Input: part model. Units: mm. Frame: model coordinates. Coordinates: 2 decimals unless noted, no trailing zeros. Write each loop counter-clockwise with the first axis right and the second up, starting at its lowest first coordinate (ties: lowest second). Pieces come first, ordered by that corner, then holes. Notation, with made-up numbers: (49, -37) -> (93, -37) arc R31 ccw to (93, -1) -> close; hole circle Ø2 at (76.5, -26). An arc over 180 degrees is marked (long way). Use one line per item in the form item = value. Start each with the question number.
(1) Cut plane C-C on y = 17. Return the cut outline in (x, z), plus the area to 3 significant figures.
(2) Cut plane A-A on x = 0. Return the cut outline in (y, z).
(3) Pull-direction query (X, two-part tool) for faces 1 (the face through (-26, 31.75, 2)), 2 (the face through (7.629, 15.653, 24.227)), 3 (the face through (10.48, 15.65, 33.29)); classes: released by +X, released by -X, zero draft, split by the parting line, or undercut.
(4) Ray query, line 1 along Y through (x, z) = (0, 28.75); line 2 along X through (y, z) = (18, -1); line 3 along X through (y, z) = (22, -17). Return the intervals inside material, ascending.
(5) Cut plane D-D on x = -17.5. Return the cut outline in (y, z).
(6) Cut plane B-B on z = 2.5. Return the cut outline in (x, y), plus the area to 3 significant figures.
(7) First-contact query: pin 1 (3 mm diameter, centred on x = -24.5, y = 21.5, fed in from -Z); pin 2 (1.5 mm diameter, centred on y = 19, z = -9, fed in from +X); pin 3 (5 mm diameter, centred on x = 0, y = 15.875, fed in from +Z) (1 decimal); pin 4 (5 mm diameter, centred on x = -21.5, y = 18.5, fed in from +Z). Flat tips, straight axial feed; report the tip coordinate or a pass-through.
```python
from build123d import *

# Parameters (mm, degrees)
SKETCH1_R                        = 34.8996
SKETCH1_R_2                      = 25.4
BOSS_EXTRUDE1_DEPTH              = 31.75
TAP_DRILL_FOR_3_8_16_TAP1_REACH  = 86.249
TAP_DRILL_FOR_3_8_16_TAP1_BORE_R = 3.96875
CIRPATTERN2_COUNT                = 6


with BuildPart() as part:
    # Sketch1 → Boss-Extrude1 (new body)
    with BuildSketch(Plane(origin=(0, 0, 0), x_dir=(1, 0, 0), z_dir=(0, 1, 0))):
        with Locations(Location((0, 0, 0), (0, 0, 270))):
            Circle(SKETCH1_R)
        with Locations(Location((0, 0, 0), (0, 0, 270))):
            Circle(SKETCH1_R_2, mode=Mode.SUBTRACT)
    extrude(amount=BOSS_EXTRUDE1_DEPTH)

    # Tap Drill for 3/8-16 Tap1 bore → Tap Drill for 3/8-16 Tap1 (cut, up to next)
    with BuildSketch(Plane.XY.offset(34.8996), mode=Mode.PRIVATE) as tap_drill_for_3_8_16_tap1_sk1:
        with Locations((0, 15.875)):
            Circle(TAP_DRILL_FOR_3_8_16_TAP1_BORE_R)
    tap_drill_for_3_8_16_tap1_tool1 = extrude(tap_drill_for_3_8_16_tap1_sk1.sketch, amount=-TAP_DRILL_FOR_3_8_16_TAP1_REACH, mode=Mode.PRIVATE) & part.part
    tap_drill_for_3_8_16_tap1 = tap_drill_for_3_8_16_tap1_tool1.solids().sort_by_distance((0, 15.875, 34.8996))[0]
    add(tap_drill_for_3_8_16_tap1, mode=Mode.SUBTRACT)

    # CirPattern2: Tap Drill for 3/8-16 Tap1 ×6 about axis
    cirpattern2_axis = Axis((0, 31.75, 0), (0, -1, 0))
    for i in range(1, CIRPATTERN2_COUNT):
        add(tap_drill_for_3_8_16_tap1.rotate(cirpattern2_axis, i * 360 / CIRPATTERN2_COUNT), mode=Mode.SUBTRACT)


solid = part.part
```
Values:
q1.outline = (-31.95, -14.05) -> (-23.65, -9.26) arc R25.4 cw to (-23.65, 9.26) -> (-31.95, 14.05) arc R34.9 ccw to start; (-28.14, -20.64) arc R34.9 ccw to (-3.81, -34.69) -> (-3.81, -25.11) arc R25.4 cw to (-19.85, -15.85) -> close; (-28.14, 20.64) -> (-19.85, 15.85) arc R25.4 cw to (-3.81, 25.11) -> (-3.81, 34.69) arc R34.9 ccw to start; (3.81, -34.69) arc R34.9 ccw to (28.14, -20.64) -> (19.85, -15.85) arc R25.4 cw to (3.81, -25.11) -> close; (3.81, 25.11) arc R25.4 cw to (19.85, 15.85) -> (28.14, 20.64) arc R34.9 ccw to (3.81, 34.69) -> close; (23.65, -9.26) -> (31.95, -14.05) arc R34.9 ccw to (31.95, 14.05) -> (23.65, 9.26) arc R25.4 cw to start
q1.area = 1,360 mm2
q2.outline = (0, -34.9) -> (11.91, -34.9) -> (11.91, -25.4) -> (0, -25.4) -> close; (0, 25.4) -> (11.91, 25.4) -> (11.91, 34.9) -> (0, 34.9) -> close; (19.84, -34.9) -> (31.75, -34.9) -> (31.75, -25.4) -> (19.84, -25.4) -> close; (19.84, 25.4) -> (31.75, 25.4) -> (31.75, 34.9) -> (19.84, 34.9) -> close
q3.face_1 = zero draft
q3.face_2 = undercut
q3.face_3 = split by the parting line
q4.line_1 = 0 to 11.91, 19.84 to 31.75
q4.line_2 = -34.89 to -25.38, 25.38 to 34.89
q4.line_3 = -30.48 to -18.87, 18.87 to 30.48
q5.outline = (0, -30.19) -> (31.75, -30.19) -> (31.75, -18.41) -> (0, -18.41) -> close; (0, 18.41) -> (31.75, 18.41) -> (31.75, 30.19) -> (0, 30.19) -> close
q6.outline = (-34.81, 0) -> (-25.28, 0) -> (-25.28, 31.75) -> (-34.81, 31.75) -> close; (25.28, 0) -> (34.81, 0) -> (34.81, 31.75) -> (25.28, 31.75) -> close
q6.area = 605 mm2
q7.pin_1 = -26.25
q7.pin_2 = 33.91
q7.pin_3 = through
q7.pin_4 = 29.27
